Verification items for this drawing (mm, ordinates from the low corner). A direction names the side the tool comes from. Round coordinates to 2 decimals unless told otherwise and drop trailing zeros. Order: outer loops, then holes, each group sorted by start corner. A loop starts at its lowest first (then second) coordinate and runs counter-clockwise, first axis right, second up. Notation, with made-up numbers: M -37.75,45 L 8.25,45 A15 cw 8.25,66 Z; hole C 69,84.25 d2. An arc over 180 degrees is marked long. Return JSON: item names as keys, results as strings. Group by question number.
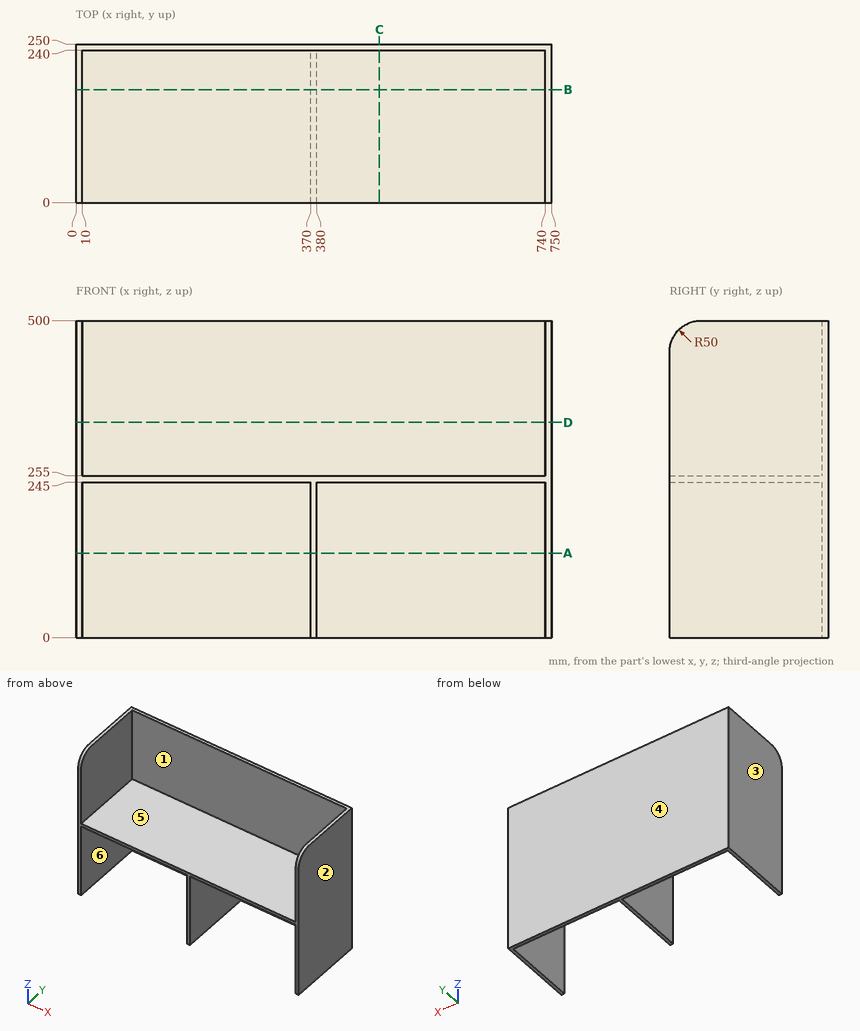
Q1. Material ranges on line 1 along X through (y, z) = (133.5, 186); line 2 along X through (y, z) = (106, 376); line 3 along Z through (x, y) = (564, 129), recorded low to high.
Q2. Section check B-B on y = 178. Record the cut outline in (x, z), plus the area to 4 significant figures.
Q3. Section check D-D on z = 339.5. Record the cut outline in (x, y).
Q4. Depth check by flat-ended pin: pin 1 Ø1.5 at (y, z) = (59.5, 65) entering from -X; pin 2 Ø1 at (x, y) = (484.5, 179.5) entering from +Z; pin 3 Ø1.5 at (x, z) = (176.5, 168) entering from -Y; pin 4 Ø12 at (x, y) = (405, 210.5) entering from -Z. Enter the tip coordinate at first touch or a pass-through.
Q5. Section check C-C on x = 478.5. Record the cut outline in (y, z).
Q6. Set-up check for the marked faces 4, 5 and 6: record each of +Z, -Z, +X, -X, +Y, -Y from which the full face is reachable in a straight line by a thin tool's end or side.
Q7. Section check A-A on z = 133. Record the cut outline in (x, y).
Q8. Release check for a two-part mould opening along X. For the marked faces 1, 2 and 3 record: +X half, -X half, draft (parallel to the pull), parting line (faces both ways), or undercut.
Geometry check:
{
 "1": {"line 1": "x = 0 to 10, 370 to 380, 740 to 750", "line 2": "x = 0 to 10, 740 to 750", "line 3": "z = 245 to 255"},
 "2": {"outline": "M 0,0 L 10,0 L 10,245 L 370,245 L 370,0 L 380,0 L 380,245 L 740,245 L 740,0 L 750,0 L 750,500 L 740,500 L 740,255 L 10,255 L 10,500 L 0,500 Z", "area": "19,750 mm^2"},
 "3": {"outline": "M 0,0 L 10,0 L 10,240 L 740,240 L 740,0 L 750,0 L 750,250 L 0,250 Z"},
 "4": {"pin 1": "stops at x = 0", "pin 2": "stops at z = 255", "pin 3": "stops at y = 240", "pin 4": "stops at z = 245"},
 "5": {"outline": "M 0,245 L 240,245 L 240,0 L 250,0 L 250,500 L 240,500 L 240,255 L 0,255 Z"},
 "6": {"face 4": "+Z, -Z, +X, -X, +Y", "face 5": "+Z, -Y", "face 6": "-Z, -Y"},
 "7": {"outline": "M 0,0 L 10,0 L 10,240 L 370,240 L 370,0 L 380,0 L 380,240 L 740,240 L 740,0 L 750,0 L 750,250 L 0,250 Z"},
 "8": {"face 1": "undercut", "face 2": "+X half", "face 3": "-X half"}
}
